Verification items for the finished model (mm, model axes). A direction names the side the tool comes from. Coordinates: 2 decimals unless noted, no trailing zeros. Write each loop counter-clockwise with the first axis right and the second up, starting at its lowest first coordinate (ties: lowest second). Pieces come first, ordered by that corner, then holes. Notation, with made-up numbers: (-20, 9) -> (28, 9) arc R37 ccw to (28, 48) -> close; hole circle Ø3 at (39, 66). An arc over 180 degrees is marked (long way). Answer in a Markdown table with one row per item.
```python
from build123d import *
from OCP.BRepFilletAPI import BRepFilletAPI_MakeChamfer

# Parameters (mm, degrees)
SKETCH2_W           = 64
SKETCH2_H           = 200
BOSS_EXTRUDE1_DEPTH = 3
SKETCH13_W          = 3
SKETCH13_H          = 40
BOSS_EXTRUDE2_DEPTH = 200
CHAMFER1_SIZE       = 1.5
CHAMFER2_SIZE       = 3
CUT_EXTRUDE1_REACH  = 129.55
SKETCH14_W          = 119
SKETCH14_H          = 37
CHAMFER3_SIZE       = 8.660254038
CHAMFER3_SIZE_2     = 5
CHAMFER4_SIZE       = 3


with BuildPart() as part:
    # Sketch2 → Boss-Extrude1 (new body)
    with BuildSketch(Plane(origin=(0, 0, 0), x_dir=(1, 0, 0), z_dir=(0, 1, 0))):
        Rectangle(SKETCH2_W, SKETCH2_H)
    extrude(amount=BOSS_EXTRUDE1_DEPTH)

    # Sketch13 → Boss-Extrude2 (add)
    with BuildSketch(Plane.XY.offset(100)):
        with Locations((33.5, -17)):
            Rectangle(SKETCH13_W, SKETCH13_H)
        with Locations((-33.5, -17)):
            Rectangle(SKETCH13_W, SKETCH13_H)
    extrude(amount=-BOSS_EXTRUDE2_DEPTH)

    # Chamfer1
    chamfer1_edges = [part.edges().sort_by_distance(p)[0] for p in [
        (-32, 0, 0),
        (32, 0, 0),
    ]]
    chamfer(chamfer1_edges, length=CHAMFER1_SIZE)

    # Chamfer2
    chamfer2_edges = [part.edges().sort_by_distance(p)[0] for p in [
        (35, 3, 0),
        (-35, 3, 0),
    ]]
    chamfer(chamfer2_edges, length=CHAMFER2_SIZE)

    # Cut-Extrude1: up to this face of the body (flat: up to its plane)
    cut_extrude1_end = Plane(part.part.faces().sort_by_distance((-35, -18.5, 0))[0])
    # Sketch14 → Cut-Extrude1 (cut, up to the picked face)
    with BuildSketch(Plane(origin=(35, 0, 0), x_dir=(0, 0, -1), z_dir=(1, 0, 0)), mode=Mode.PRIVATE) as cut_extrude1_sk1:
        with Locations((0, -18.5)):
            Rectangle(SKETCH14_W, SKETCH14_H)
    cut_extrude1_tool1 = split(extrude(cut_extrude1_sk1.sketch, amount=-CUT_EXTRUDE1_REACH, mode=Mode.PRIVATE), bisect_by=cut_extrude1_end, keep=Keep.BOTH, mode=Mode.PRIVATE)
    add(cut_extrude1_tool1.solids().sort_by(Axis((35, -18.5, 0), (-1, 0, 0)))[0], mode=Mode.SUBTRACT)

    # Chamfer3
    chamfer3_edges_1 = [part.edges().sort_by_distance(p)[0] for p in [
        (32.75, 0, -59.5),
    ]]
    chamfer3_side_1 = [part.faces().sort_by_distance(p)[0] for p in [
        (32.75, 0, -59.4),
    ]]
    chamfer3_edges_2 = [part.edges().sort_by_distance(p)[0] for p in [
        (-32.75, 0, -59.5),
    ]]
    chamfer3_side_2 = [part.faces().sort_by_distance(p)[0] for p in [
        (-32.75, 0, -59.4),
    ]]
    chamfer3_edges_3 = [part.edges().sort_by_distance(p)[0] for p in [
        (32.75, 0, 59.5),
    ]]
    chamfer3_side_3 = [part.faces().sort_by_distance(p)[0] for p in [
        (32.75, 0, 59.4),
    ]]
    chamfer3_edges_4 = [part.edges().sort_by_distance(p)[0] for p in [
        (-32.75, 0, 59.5),
    ]]
    chamfer3_side_4 = [part.faces().sort_by_distance(p)[0] for p in [
        (-32.75, 0, 59.4),
    ]]
    chamfer3 = BRepFilletAPI_MakeChamfer(part.part.solid().wrapped)
    for e in chamfer3_edges_1:
        chamfer3.Add(CHAMFER3_SIZE - 0.0001, CHAMFER3_SIZE_2 - 0.0001, e.wrapped, chamfer3_side_1[0].wrapped)
    for e in chamfer3_edges_2:
        chamfer3.Add(CHAMFER3_SIZE - 0.0001, CHAMFER3_SIZE_2 - 0.0001, e.wrapped, chamfer3_side_2[0].wrapped)
    for e in chamfer3_edges_3:
        chamfer3.Add(CHAMFER3_SIZE - 0.0001, CHAMFER3_SIZE_2 - 0.0001, e.wrapped, chamfer3_side_3[0].wrapped)
    for e in chamfer3_edges_4:
        chamfer3.Add(CHAMFER3_SIZE - 0.0001, CHAMFER3_SIZE_2 - 0.0001, e.wrapped, chamfer3_side_4[0].wrapped)
    add(Compound.cast(chamfer3.Shape()), mode=Mode.REPLACE)  # a hair under: the kernel refuses the full size

    # Chamfer4
    chamfer4_edges = [part.edges().sort_by_distance(p)[0] for p in [
        (33.5, -37, 100),
        (33.5, -37, -100),
        (-33.5, -37, 100),
        (-33.5, -37, -100),
        (33.5, -37, -59.5),
        (-33.5, -37, 59.5),
        (-33.5, -37, -59.5),
        (33.5, -37, 59.5),
    ]]
    chamfer(chamfer4_edges, length=CHAMFER4_SIZE)


solid = part.part
```
1. Section check A-A, the plane y = -12. Record the boundary of the cut face in (x, z).
Geometry says:
| item | result |
|---|---|
| outline | (-35, -100) -> (-32, -100) -> (-32, -59.5) -> (-35, -59.5) -> close; (-35, 59.5) -> (-32, 59.5) -> (-32, 100) -> (-35, 100) -> close; (32, -100) -> (35, -100) -> (35, -59.5) -> (32, -59.5) -> close; (32, 59.5) -> (35, 59.5) -> (35, 100) -> (32, 100) -> close |
2. Section check D-D, the plane z = -57. Record the boundary of the cut face in (x, y), plus the area to 3 significant figures.
Geometry says:
| item | result |
|---|---|
| outline | (-35, -3.56) -> (-32, -3.56) -> (-32, -1.5) -> (-30.5, 0) -> (30.5, 0) -> (32, -1.5) -> (32, -3.56) -> (35, -3.56) -> (35, 0) -> (32, 3) -> (-32, 3) -> (-35, 0) -> close |
| area | 225 mm^2 |
3. Section check B-B, the plane z = 70.5. Record the boundary of the cut face in (x, y), plus the area to 3 significant figures.
Geometry says:
| item | result |
|---|---|
| outline | (-35, -37) -> (-32, -37) -> (-32, -1.5) -> (-30.5, 0) -> (30.5, 0) -> (32, -1.5) -> (32, -37) -> (35, -37) -> (35, 0) -> (32, 3) -> (-32, 3) -> (-35, 0) -> close |
| area | 425 mm^2 |
4. Depth check by flat-ended pin: P1, Ø21, axis at x = -6, z = 8, coming from the -Y side. Enter the tip coordinate at first touch or a pass-through.
Geometry says:
| item | result |
|---|---|
| P1 | y = 0 |
5. Section check C-C, the plane x = -13. Record the boundary of the cut face in (y, z).
Geometry says:
| item | result |
|---|---|
| outline | (0, -100) -> (3, -100) -> (3, 100) -> (0, 100) -> close |
6. Thickness scan on line 1 (X direction, y = -27, z = 87.5); line 2 (Y direction, x = 12, z = -10). Record the ranges inside material, lowest first. Write a range as from..to.
Geometry says:
| item | result |
|---|---|
| line 1 | -35..-32, 32..35 |
| line 2 | 0..3 |
7. Tool access check on faces 1 (the flat face through (35, -19, -81)), 2 (the flat face through (32, -19, -82)), 3 (the flat face through (33.281, -2.535, 55.231)). Record the directions out of +Z, -Z, +X, -X, +Y, -Y that give a thin tool (end or side, any length) a straight path to the whole face; none if there is none.
Geometry says:
| item | result |
|---|---|
| face 1 | +Z, -Z, +X, +Y, -Y |
| face 2 | +Z, -Z, -Y |
| face 3 | +X, -X, -Y |
8. Mould release check, pull along X, two halves, no side actions. Record for faces 4 (the flat face through (0, 0, -1)), 5 (the flat face through (-3, 1, -100)), 6 (the flat face through (-35, -19, -81)): released by +X, released by -X, zero draft, split by the parting line, or undercut.
Geometry says:
| item | result |
|---|---|
| face 4 | undercut |
| face 5 | zero draft |
| face 6 | released by -X |
